```python
from build123d import *

# Parameters (mm, degrees)
SKETCH1_R           = 2.8
BOSS_EXTRUDE1_DEPTH = 3.2
CUT_EXTRUDE1_DEPTH  = 2.2
SKETCH3_R           = 0.75
CUT_EXTRUDE2_DEPTH  = 1
BOSS_EXTRUDE2_DEPTH = 1
CUT_EXTRUDE3_REACH  = 5.2
SKETCH5_R           = 0.5


with BuildPart() as part:
    # Sketch1 → Boss-Extrude1 (new body)
    with BuildSketch(Plane.XY):
        Circle(SKETCH1_R)
    extrude(amount=BOSS_EXTRUDE1_DEPTH)

    # Sketch2 → Cut-Extrude1 (cut)
    with BuildSketch(Plane.XY.offset(3.2)):
        Polygon((0.014651949, 1.985348051), (-0.313876209, 1.636970634), (-0.750714916, 1.833107116), (-0.920917091, 1.385526068), (-1.399561614, 1.399561614), (-1.385526068, 0.920917091), (-1.833107116, 0.750714916), (-1.636970634, 0.313876209), (-1.985348051, -0.014651949), (-1.636970634, -0.343180107), (-1.833107116, -0.780018813), (-1.385526068, -0.950220989), (-1.399561614, -1.428865511), (-0.920917091, -1.414829965), (-0.750714916, -1.862411014), (-0.313876209, -1.666274532), (0.014651949, -2.014651949), (0.343180107, -1.666274532), (0.780018813, -1.862411014), (0.950220989, -1.414829965), (1.428865511, -1.428865511), (1.414829965, -0.950220989), (1.862411014, -0.780018813), (1.666274532, -0.343180107), (2.014651949, -0.014651949), (1.666274532, 0.313876209), (1.862411014, 0.750714916), (1.414829965, 0.920917091), (1.428865511, 1.399561614), (0.950220989, 1.385526068), (0.780018813, 1.833107116), (0.343180107, 1.636970634), align=None)
    extrude(amount=-CUT_EXTRUDE1_DEPTH, mode=Mode.SUBTRACT)

    # Sketch3 → Cut-Extrude2 (cut)
    with BuildSketch(Plane.XY):
        Circle(SKETCH3_R)
    extrude(amount=CUT_EXTRUDE2_DEPTH, mode=Mode.SUBTRACT)

    # Sketch4 → Boss-Extrude2 (add)
    with BuildSketch(Plane.XY):
        with BuildLine():
            ThreePointArc((10.15, 1.85), (12, 0), (10.15, -1.85))
            Line((10.15, -1.85), (0.75, -1.85))
            Line((0.75, -1.85), (0.75, 1.85))
            Line((0.75, 1.85), (10.15, 1.85))
        make_face()
        with BuildLine():
            Line((-0.75, 1.85), (-10.15, 1.85))
            ThreePointArc((-10.15, 1.85), (-12, 0), (-10.15, -1.85))
            Line((-10.15, -1.85), (-0.75, -1.85))
            Line((-0.75, -1.85), (-0.75, 1.85))
        make_face()
    extrude(amount=BOSS_EXTRUDE2_DEPTH)

    # Sketch5 → Cut-Extrude3 (cut, up to next)
    with BuildSketch(Plane(origin=(0, 0, 0), x_dir=(-1, 0, 0), z_dir=(0, 0, -1)), mode=Mode.PRIVATE) as cut_extrude3_sk1:
        with Locations((10, 0)):
            Circle(SKETCH5_R)
    cut_extrude3_tool1 = extrude(cut_extrude3_sk1.sketch, amount=-CUT_EXTRUDE3_REACH, mode=Mode.PRIVATE) & part.part
    add(cut_extrude3_tool1.solids().sort_by_distance((-10, 0, 0))[0], mode=Mode.SUBTRACT)
    # Sketch5 → Cut-Extrude3 (cut, up to next)
    with BuildSketch(Plane(origin=(0, 0, 0), x_dir=(-1, 0, 0), z_dir=(0, 0, -1)), mode=Mode.PRIVATE) as cut_extrude3_sk2:
        with Locations((-10, 0)):
            Circle(SKETCH5_R)
    cut_extrude3_tool2 = extrude(cut_extrude3_sk2.sketch, amount=-CUT_EXTRUDE3_REACH, mode=Mode.PRIVATE) & part.part
    add(cut_extrude3_tool2.solids().sort_by_distance((10, 0, 0))[0], mode=Mode.SUBTRACT)


solid = part.part
```
Input: part model. Units: mm. Frame: model coordinates. A direction names the side the tool comes from. Coordinates: 2 decimals unless noted, no trailing zeros. Write each loop counter-clockwise with the first axis right and the second up, starting at its lowest first coordinate (ties: lowest second). Pieces come first, ordered by that corner, then holes. Notation, with made-up numbers: (-5.5, 46) -> (4.5, 46) arc R25 cw to (4.5, 84) -> close; hole circle Ø7 at (16.25, 27.25). An arc over 180 degrees is marked (long way). Answer as a JSON object with one key per item and string values.
1. Mould query, pull axis Y, two halves, no side actions, for faces 4 (the face through (1, -2, 3.2)), 5 (the face through (-0.365, 2.776, 1.933)), 6 (the face through (-0.75, 0.03, 0.49)). Classes: released by +Y, released by -Y, zero draft, split by the parting line, or undercut.
Result set:
{"face 4": "zero draft", "face 5": "split by the parting line", "face 6": "undercut"}
2. Section C-C on x = -5. Return the cut outline in (y, z).
Result set:
{"outline": "(-1.85, 0) -> (1.85, 0) -> (1.85, 1) -> (-1.85, 1) -> close"}
3. Access query for faces 1 (the face through (-1, 0, 1)), 2 (the face through (6.1, 1.85, 0.5)), 3 (the face through (-6.1, 1.85, 0.5)). Directions: +Z, -Z, +X, -X, +Y, -Y. A direction counts if a zero-diameter tool reaches every point of the face in a straight line with its end or side. Return the directions, or none.
Result set:
{"face 1": "+Z", "face 2": "+Z, -Z, +X, +Y", "face 3": "+Z, -Z, -X, +Y"}
4. First-contact query: P1, Ø2, axis at x = 0, y = 0, coming from the +Z side; P2, Ø1.1, axis at x = -7, z = 0.5, coming from the +Y side; P3, Ø0.5, axis at x = -5, z = 0.5, coming from the -Y side. Flat tips, straight axial feed; report the tip coordinate or a pass-through.
Result set:
{"P1": "stops at z = 1", "P2": "stops at y = 1.85", "P3": "stops at y = -1.85"}
5. Material intervals for line 1 (Y direction, x = -10, z = 0.65); line 2 (Y direction, x = 0, z = 0.4); line 3 (X direction, y = 0.6, z = 0.6), sorted ascending. Write a range as from..to.
Result set:
{"line 1": "y = -1.85..-0.5, 0.5..1.85", "line 2": "y = -2.8..-0.75, 0.75..2.8", "line 3": "x = -11.9..-0.45, 0.45..11.9"}
6. Section A-A on z = 0.55. Return the cut outline in (x, y).
Result set:
{"outline": "(-10.15, -1.85) -> (-2.1, -1.85) arc R2.8 ccw to (2.1, -1.85) -> (10.15, -1.85) arc R1.85 ccw to (10.15, 1.85) -> (2.1, 1.85) arc R2.8 ccw to (-2.1, 1.85) -> (-10.15, 1.85) arc R1.85 ccw to start; hole circle Ø1 at (-10, 0); hole circle Ø1.5 at (0, 0); hole circle Ø1 at (10, 0)"}
7. Section D-D on y = 2.4. Return the cut outline in (x, z), then the cut area to 3 significant figures.
Result set:
{"outline": "(-1.44, 0) -> (1.44, 0) -> (1.44, 3.2) -> (-1.44, 3.2) -> close", "area": "9.23 mm2"}
